Autodesk Inventor part; units mm, degrees
ref_plane "Arbeitsebene1" through (-5.2721, -5.2721, 15) normal (0.7071, -0.7071, 0) x (-0.7071, -0.7071, 0)
ref_plane "Arbeitsebene2" through (-18, -7.4558, 15) normal (0.3827, -0.9239, 0) x (0, 0, -1)
ref_plane "Arbeitsebene3" through (0, -18, 15) normal (1, 0, 0) x (0, 1, 0)
sketch "Skizze1" plane through (0, 0, 0) normal (0, 0, 1) x (1, 0, 0)
  line L0 (-8.2843, 20) -> (8.2843, 20)
  line L1 (8.2843, 20) -> (20, 8.2843)
  line L2 (20, 8.2843) -> (20, -8.2843)
  line L3 (20, -8.2843) -> (8.2843, -20)
  line L4 (8.2843, -20) -> (-8.2843, -20)
  line L5 (-8.2843, -20) -> (-20, -8.2843)
  line L6 (-20, -8.2843) -> (-20, 8.2843)
  line L7 (-20, 8.2843) -> (-8.2843, 20)
  line L8 (0, -28) -> (0, 28)
  line L9 (-28, 0) -> (28, 0)
  point P0 (0, 0)
  dimension "d0" = 40
  dimension "d1" = 40
extrude "Extrusion1" add sketch "Skizze1" along normal blind 15
sketch "Skizze2" plane through (0, 0, 15) normal (0, 0, 1) x (1, 0, 0)
  line L0 (8.2843, 20) -> (-8.2843, 20)
  line L1 (-8.2843, 20) -> (-20, 8.2843)
  line L2 (-20, 8.2843) -> (-20, -8.2843)
  line L3 (-20, -8.2843) -> (-8.2843, -20)
  line L4 (-8.2843, -20) -> (8.2843, -20)
  line L5 (8.2843, -20) -> (20, -8.2843)
  line L6 (20, -8.2843) -> (20, 8.2843)
  line L7 (20, 8.2843) -> (8.2843, 20)
  line L8 (-7.4558, 18) -> (7.4558, 18)
  line L9 (7.4558, 18) -> (18, 7.4558)
  line L10 (18, 7.4558) -> (18, -7.4558)
  line L11 (18, -7.4558) -> (7.4558, -18)
  line L12 (7.4558, -18) -> (-7.4558, -18)
  line L13 (-7.4558, -18) -> (-18, -7.4558)
  line L14 (-18, -7.4558) -> (-18, 7.4558)
  line L15 (-18, 7.4558) -> (-7.4558, 18)
  point P0 (0, 0)
  dimension "d4" = 2
extrude "Extrusion2" cut sketch "Skizze2" against normal blind 12 contours L8 L9 L10 L11 L12 L13 L14 L15
sketch "Skizze3" plane through (-18, -7.4558, 15) normal (1, 0, 0) x (0, 0, -1)
  line L0 (0, 0) -> (0, 14.9117)
  line L1 (0, 0) -> (12, 0)
  line L2 (12, 0) -> (12, 14.9117)
  line L3 (0, 14.9117) -> (12, 14.9117)
  line L4 (12, 0) -> (12, 14.9117)
  line L5 (12, 7.4558) -> (0, 7.4558)
  line L6 (0, 0) -> (0, 14.9117)
  point P0 (15, 7.4558)
  point P1 (8, 9.4558)
  point P2 (8, 5.4558)
  dimension "d7" = 4
  dimension "d23" = 4
hole "Bohrung1" at (-18, 2, 7) at (-18, -2, 7) direction (-1, 0, 0) diameter 2.2 end through all
mirror "Spiegeln1" about plane through (0, 0, 0) normal (1, 0, 0) of "Bohrung1"
ref_plane "Arbeitsebene1" through (-5.2721, -5.2721, 15) normal (0.7071, -0.7071, 0) x (-0.7071, -0.7071, 0)
mirror "Spiegeln2" about plane through (-5.2721, -5.2721, 15) normal (0.7071, -0.7071, 0) of "Bohrung1"
sketch "Skizze4" plane through (-7.4558, -18, 3) normal (0.7071, 0.7071, 0) x (-0.7071, 0.7071, 0)
  point P0 (7.4558, -3)
ref_plane "Arbeitsebene2" through (-18, -7.4558, 15) normal (0.3827, -0.9239, 0) x (0, 0, -1)
mirror "Spiegeln3" about plane through (-18, -7.4558, 15) normal (0.3827, -0.9239, 0) of "Bohrung1"
mirror "Spiegeln4" about plane through (0, 0, 0) normal (0, 1, 0) of "Bohrung1", "Spiegeln2"
mirror "Spiegeln5" about plane through (0, 0, 0) normal (1, 0, 0) of "Bohrung1", "Spiegeln3"
mirror "Spiegeln6" about plane through (0, 0, 0) normal (0, 1, 0) of "Bohrung1", "Spiegeln3", "Spiegeln5"
sketch "Skizze6" plane through (-8.2843, -20, 15) normal (-0.7071, -0.7071, 0) x (-0.7071, 0.7071, 0)
  circle A0 centre (4.2843, 3.0841) radius 2.3005
  circle A1 centre (6.2843, 8) radius 1.1
  circle A2 centre (10.2843, 8) radius 1.1
  line L0 (0, 15) -> (16.5685, 15)
  line L1 (0, 15) -> (0, 0)
  line L2 (16.5685, 0) -> (0, 0)
  line L3 (16.5685, 15) -> (16.5685, 0)
  circle A3 centre (12.2843, 3.0841) radius 2.3005
  line L4 (8.2843, 15) -> (8.2843, 0)
  line L5 (16.5685, 0) -> (0, 0)
  dimension "d24" = 4.601
  dimension "d25" = 4.601
  dimension "d26" = 8
extrude "Extrusion3" add sketch "Skizze6" along normal blind 1.8 contours A0 | A3
chamfer "Fase1" distance 0.135 angle 45 2 edges at (-10.9598, -19.8701, 11.9159) (-16.6167, -14.2132, 11.9159)
sketch "Skizze7" plane through (8.2843, 20, 0) normal (0.7071, 0.7071, 0) x (-0.7071, 0.7071, 0)
  circle A0 centre (-4.2843, 11.9159) radius 2.3005
  circle A1 centre (-12.2843, 11.9159) radius 2.3005
  circle A2 centre (-4.2843, 11.9159) radius 2.3985
  circle A3 centre (-12.2843, 11.9159) radius 2.3985
  point P0 (-8.2843, 0)
  dimension "d33" = 4.797
  dimension "d34" = 4.797
extrude "Extrusion4" cut sketch "Skizze7" against normal blind 2.2 contours A0 | A1 | A2 | A3
sketch "Skizze8" plane through (0, 0, 0) normal (0, 0, -1) x (-1, 0, 0)
  line L0 (8.2843, 20) -> (-8.2843, 20)
  line L1 (-8.2843, 20) -> (-20, 8.2843)
  line L2 (-20, 8.2843) -> (-20, -8.2843)
  line L3 (-20, -8.2843) -> (-8.2843, -20)
  line L4 (-8.2843, -20) -> (8.2843, -20)
  line L5 (8.2843, -20) -> (20, -8.2843)
  line L6 (20, -8.2843) -> (20, 8.2843)
  line L7 (20, 8.2843) -> (8.2843, 20)
  line L8 (8.2843, -20) -> (20, -8.2843)
  line L9 (14.1421, -14.1421) -> (-14.1421, 14.1421)
  line L10 (-20, 8.2843) -> (-8.2843, 20)
  point P0 (0, 0)
  point P1 (1.0607, -1.0607)
  point P2 (-1.0607, 1.0607)
  dimension "d43" = 3
  dimension "d44" = 1.5
hole "Bohrung3" at (-1.0607, -1.0607, 0) at (1.0607, 1.0607, 0) direction (0, 0, 1) diameter 1.8 end through all
ref_plane "Arbeitsebene3" through (0, -18, 15) normal (1, 0, 0) x (0, 1, 0)
mirror "Spiegeln7" about plane through (0, -18, 15) normal (1, 0, 0) of "Extrusion3", "Extrusion4"
sketch "Skizze9" plane through (0, 0, 0) normal (0, 0, -1) x (-1, 0, 0)
  circle A0 centre (1.0607, -1.0607) radius 0.9
  circle A1 centre (-1.0607, 1.0607) radius 0.9
  line L0 (8.2843, 20) -> (-8.2843, 20)
  line L1 (-8.2843, 20) -> (-20, 8.2843)
  line L2 (-20, 8.2843) -> (-20, -8.2843)
  line L3 (-20, -8.2843) -> (-8.2843, -20)
  line L4 (-8.2843, -20) -> (8.2843, -20)
  line L5 (8.2843, -20) -> (20, -8.2843)
  line L6 (20, -8.2843) -> (20, 8.2843)
  line L7 (20, 8.2843) -> (8.2843, 20)
  line L8 (7.0004, 12.7986) -> (7.0004, 12.7986)
  line L9 (7.0004, 11.243) -> (11.243, 7.0004)
  line L10 (12.7986, 7.0004) -> (12.7986, 7.0004)
  line L11 (12.7986, 8.556) -> (8.556, 12.7986)
  line L12 (20, 8.2843) -> (8.2843, 20)
  line L13 (0, 0) -> (14.1421, 14.1421)
  arc A2 (11.243, 7.0004) -> (12.7986, 7.0004) centre (12.0208, 7.7782) ccw
  arc A3 (12.7986, 7.0004) -> (12.7986, 8.556) centre (12.0208, 7.7782) ccw
  arc A4 (7.0004, 12.7986) -> (7.0004, 11.243) centre (7.7782, 12.0208) ccw
  arc A5 (8.556, 12.7986) -> (7.0004, 12.7986) centre (7.7782, 12.0208) ccw
  dimension "d52" = 1.1
  dimension "d53" = 1.1
  dimension "d54" = 2.2
  dimension "d55" = 3
  dimension "d58" = 6
extrude "Extrusion5" cut sketch "Skizze9" along normal mid plane 10 contours L11 A3 A2 L9 L13 | L13 L9 A4 A5 L11
equation "\"d1\" = d0"
equation "\"d34\" = d33"
properties part number "oktagonOben_v2"
Geometry check sheet. Reference: the model listing, model coordinates, mm. A direction names the side the tool comes from. Give positions to 0.01 mm unless a question says otherwise; leave off trailing zeros. Order: outer loops, then holes, each group sorted by start corner. A loop starts at its lowest first (then second) coordinate and runs counter-clockwise, first axis right, second up.
1. Access from +Z, -Z, +X, -X, +Y, -Y to the whole of each face (thin tool, end or side, straight path). Record for faces 1 (the face through (-9.092, 9.151, 1.521)), 2 (the face through (16.494, 10.396, 14.294)), 3 (the face through (-12.802, 12.654, 9.084)).
2. Release check for a two-part mould opening along Y. For faces 4 (the face through (1.579, -19.014, 5.984)), 5 (the face through (-18.22, -12.61, 11.89)), 6 (the face through (12.802, -12.654, 9.084)) record: pulls with the +Y half, pulls with the -Y half, needs draft (parallel to the pull), parting line crosses it, or undercut.
3. Thickness scan on L1, parallel to Z at x = -18.8, y = -2; L2, parallel to X at y = 3, z = 8.5; L3, parallel to X at y = 19.05, z = 7. Record the ranges inside material, lowest first.
4. Section check D-D, the plane y = 10. Give the number of separate pieces and of enclosed holes in the cut face, and give its area (3 significant figures).
5. Section check B-B, the plane y = 4. Enter the section's corners in (x, z), and give its area (3 significant figures).
6. Section check A-A, the plane z = 3.5. Enter the section's corners in (x, y), and give its area (3 significant figures).
7. Gauge pin test, flat ends, axial feed: pin 1 Ø1.1 at (x, y) = (-1.06, -1.06) entering from +Z (1 decimal); pin 2 Ø6 at (y, z) = (11.5, 8.5) entering from +X. Record the tip position at first contact, or that the pin passes through.
Values follow:
1. face 1: +Z, -Z
1. face 2: none
1. face 3: +Z
2. face 4: needs draft
2. face 5: pulls with the -Y half
2. face 6: undercut
3. L1: z = 0 to 5.9, 8.1 to 15
3. L2: x = -20 to -18, 18 to 20
3. L3: x = -9.23 to -3.1, -0.9 to 0.9, 3.1 to 9.23
4. separate pieces: 4
4. enclosed holes: 0
4. area: 144 mm2
5. outline: (-20, 0) - (20, 0) - (20, 15) - (18, 15) - (18, 3) - (-18, 3) - (-18, 15) - (-20, 15) - close
5. area: 168 mm2
6. outline: (-20, -8.28) - (-8.28, -20) - (8.28, -20) - (20, -8.28) - (20, 8.28) - (8.28, 20) - (-8.28, 20) - (-20, 8.28) - close; hole (-18, -7.46) - (-7.46, -18) - (7.46, -18) - (18, -7.46) - (18, 7.46) - (7.46, 18) - (-7.46, 18) - (-18, 7.46) - close
6. area: 252 mm2
7. pin 1: passes through
7. pin 2: stops at x = 19.78
